```python
from build123d import *

# Parameters (mm, degrees)
F0_R     = 34.671
F1_DEPTH = 5.08
F3_DEPTH = 25.4
F4_SIZE2 = 1.778
F4_SIZE  = 1.27


with BuildPart() as f1:
    # F0 (on Top) → F1 (new body)
    with BuildSketch(Plane.XY):
        Circle(F0_R)
    extrude(amount=F1_DEPTH)

    # F2 (on face) → F3 (cut)
    with BuildSketch(Plane.XY.offset(5.08)):
        with BuildLine():
            ThreePointArc((21.1934044457, 21.1934044457), (18.8585378542, 21.1934044457), (18.8585378542, 18.8585378542))
            Line((18.8585378542, 18.8585378542), (21.1934044457, 21.1934044457))
        make_face()
        with BuildLine():
            Line((21.1934044457, 21.1934044457), (18.8585378542, 18.8585378542))
            ThreePointArc((18.8585378542, 18.8585378542), (20.6577814968, 18.5006460418), (21.67697115, 20.02597115))
            ThreePointArc((21.67697115, 20.02597115), (21.5512962582, 20.6577814968), (21.1934044457, 21.1934044457))
        make_face()
        with BuildLine():
            ThreePointArc((-18.37497115, -20.02597115), (-18.5006460418, -19.3941608031), (-18.8585378542, -18.8585378542))
            Line((-18.8585378542, -18.8585378542), (-21.1934044457, -21.1934044457))
            ThreePointArc((-21.1934044457, -21.1934044457), (-19.3941608031, -21.5512962582), (-18.37497115, -20.02597115))
        make_face()
        with BuildLine():
            Line((-21.1934044457, -21.1934044457), (-18.8585378542, -18.8585378542))
            ThreePointArc((-18.8585378542, -18.8585378542), (-21.1934044457, -18.8585378542), (-21.1934044457, -21.1934044457))
        make_face()
        with BuildLine():
            ThreePointArc((-21.1934044457, 21.1934044457), (-21.1934044457, 18.8585378542), (-18.8585378542, 18.8585378542))
            Line((-18.8585378542, 18.8585378542), (-21.1934044457, 21.1934044457))
        make_face()
        with BuildLine():
            Line((-21.1934044457, 21.1934044457), (-18.8585378542, 18.8585378542))
            ThreePointArc((-18.8585378542, 18.8585378542), (-18.5006460418, 19.3941608031), (-18.37497115, 20.02597115))
            ThreePointArc((-18.37497115, 20.02597115), (-19.3941608031, 21.5512962582), (-21.1934044457, 21.1934044457))
        make_face()
        with BuildLine():
            ThreePointArc((21.67697115, -20.02597115), (20.6577814968, -18.5006460418), (18.8585378542, -18.8585378542))
            Line((18.8585378542, -18.8585378542), (21.1934044457, -21.1934044457))
            ThreePointArc((21.1934044457, -21.1934044457), (21.5512962582, -20.6577814968), (21.67697115, -20.02597115))
        make_face()
        with BuildLine():
            Line((21.1934044457, -21.1934044457), (18.8585378542, -18.8585378542))
            ThreePointArc((18.8585378542, -18.8585378542), (18.8585378542, -21.1934044457), (21.1934044457, -21.1934044457))
        make_face()
    extrude(amount=-F3_DEPTH, mode=Mode.SUBTRACT)

    # F4
    f4_edges = [f1.edges().sort_by_distance(p)[0] for p in [
        (-21.193404, -21.193404, 0),
        (21.193404, -21.193404, 0),
        (21.193404, 21.193404, 0),
        (-21.193404, 21.193404, 0),
    ]]
    chamfer(f4_edges, length=F4_SIZE, length2=F4_SIZE2)


solid = f1.part
```
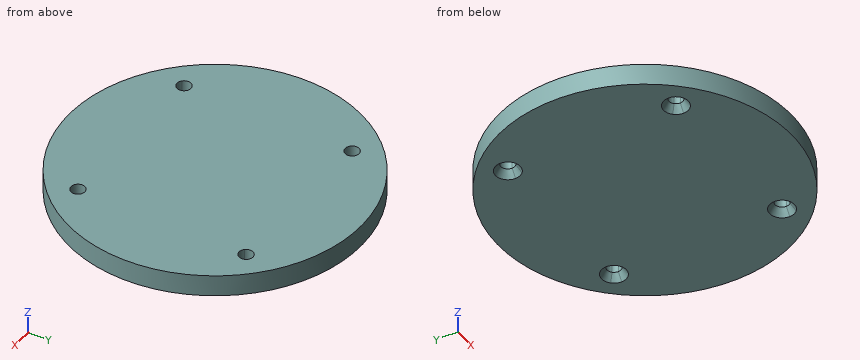
Read the model definition and answer for the solid it produces. Units are mm, in the model's axes. Give positions to 0.01 mm unless a question says otherwise; leave off trailing zeros. Loops run counter-clockwise (first coordinate to the right, second up) from the corner with the lowest first, then second, coordinate; pieces in that order, holes last.
Item 1: This flat-tipped pin is pushed along its axis until it touches: pin 1 Ø1.5 at (x, z) = (-19, 3) entering from -Y. Where does it stop, or does it pass through?
Item 2: Find the intervals of material crossed by line 1 along Y through (x, z) = (-21, 1.25); line 2 along X through (y, z) = (-19, 2.6); line 3 along Y through (x, z) = (0.5, 3), in increasing order.
Item 3: The part is cut by section B-B (x = 25). Write down the section's boundary in (y, z), and give its area (3 significant figures).
Item 4: The part is cut by section A-A (z = 3.4). Write down the section's boundary in (x, y).
Item 5: The part is cut by section C-C (y = 29). Write down the section's boundary in (x, z), and give its area (3 significant figures).
Taken from the geometry:
1. pin 1: stops at y = -29.48
2. line 1: y = -27.59 to -21.8, -18.25 to 18.25, 21.8 to 27.59
2. line 2: x = -29 to -21.32, -18.73 to 18.73, 21.32 to 29
2. line 3: y = -34.67 to 34.67
3. outline: (-24.02, 0) - (24.02, 0) - (24.02, 5.08) - (-24.02, 5.08) - close
3. area: 244 mm2
4. outline: circle Ø69.34 at (0, 0); hole circle Ø3.3 at (-20.03, -20.03); hole circle Ø3.3 at (-20.03, 20.03); hole circle Ø3.3 at (20.03, -20.03); hole circle Ø3.3 at (20.03, 20.03)
5. outline: (-19, 0) - (19, 0) - (19, 5.08) - (-19, 5.08) - close
5. area: 193 mm2
